The model under review builds one solid part; all positions refer to its coordinate system, in mm. A direction names the side the tool comes from. Round coordinates to 2 decimals unless told otherwise and drop trailing zeros. Write each loop counter-clockwise with the first axis right and the second up, starting at its lowest first coordinate (ties: lowest second). Pieces come first, ordered by that corner, then holes. Notation, with made-up numbers: (63, 32) - (112, 32) arc R26 cw to (112, 66) - close; hole circle Ø11 at (25.5, 22.5). An arc over 180 degrees is marked (long way). Return JSON: item names as keys, results as strings.
from build123d import *

# Parameters (mm, degrees)
EXTRUDE_1_DEPTH              = 25
EXTRUDE_2_DEPTH              = 10
HOLE_WIZARD_M8_1_D           = 15
HOLE_WIZARD_M8_1_CBORE_D     = 30
HOLE_WIZARD_M8_1_CBORE_DEPTH = 10
CUT_EXTRUDE_1_DEPTH          = 20
SKETCH_6_R                   = 35.5
EXTRUDE_3_DEPTH              = 130
SKETCH_7_R                   = 38.335
EXTRUDE_4_DEPTH              = 130
EXTRUDE_8_DEPTH              = 70
CUT_EXTRUDE_2_REACH          = 225
SKETCH_9_R                   = 20.5
CUT_EXTRUDE_3_REACH          = 212
SKETCH_10_R                  = 20.5
CHAMFER_1_SIZE               = 2


with BuildPart() as part:
    # Sketch 1 → Extrude 1 (new body)
    with BuildSketch(Plane(origin=(0, 0, 0), x_dir=(1, 0, 0), z_dir=(0, 1, 0))):
        with BuildLine():
            Line((10, 0), (190, 0))
            ThreePointArc((190, 0), (197.071067812, 2.928932188), (200, 10))
            Line((200, 10), (200, 203))
            ThreePointArc((200, 203), (197.071067812, 210.071067812), (190, 213))
            Line((190, 213), (10, 213))
            ThreePointArc((10, 213), (2.928932188, 210.071067812), (0, 203))
            Line((0, 203), (0, 10))
            ThreePointArc((0, 10), (2.928932188, 2.928932188), (10, 0))
        make_face()
    extrude(amount=EXTRUDE_1_DEPTH)

    # Sketch 2 → Extrude 2 (add)
    with BuildSketch(Plane(origin=(0, 25, 0), x_dir=(1, 0, 0), z_dir=(0, 1, 0))):
        with BuildLine():
            Line((140, 0), (190, 0))
            ThreePointArc((190, 0), (197.071067812, 2.928932188), (200, 10))
            Line((200, 10), (200, 60))
            Line((200, 60), (155, 60))
            ThreePointArc((155, 60), (144.393398282, 55.606601718), (140, 45))
            Line((140, 45), (140, 0))
        make_face()
    extrude(amount=EXTRUDE_2_DEPTH)

    # Hole Wizard M8 _ _ _ _1 (through all)
    with Locations(Plane(origin=(170, 35, -30), x_dir=(0, 0, 1), z_dir=(0, 1, 0))):
        with Locations((0, 0)):
            CounterBoreHole(HOLE_WIZARD_M8_1_D / 2, HOLE_WIZARD_M8_1_CBORE_D / 2, HOLE_WIZARD_M8_1_CBORE_DEPTH)

    # Sketch 5 → Cut-Extrude 1 (cut)
    with BuildSketch(Plane(origin=(0, 25, 0), x_dir=(1, 0, 0), z_dir=(0, 1, 0))):
        with BuildLine():
            Line((149.247641486, 146), (181, 146))
            ThreePointArc((181, 146), (188.071067812, 143.071067812), (191, 136))
            Line((191, 136), (191, 79))
            ThreePointArc((191, 79), (188.071067812, 71.928932188), (181, 69))
            Line((181, 69), (155, 69))
            ThreePointArc((155, 69), (138.029437252, 61.970562748), (131, 45))
            Line((131, 45), (131, 19))
            ThreePointArc((131, 19), (128.071067812, 11.928932188), (121, 9))
            Line((121, 9), (64, 9))
            ThreePointArc((64, 9), (56.928932188, 11.928932188), (54, 19))
            Line((54, 19), (54, 50.752358514))
            ThreePointArc((54, 50.752358514), (56.018165786, 56.776503481), (61.258064516, 60.369103795))
            ThreePointArc((61.258064516, 60.369103795), (110.610173055, 89.389826945), (139.630896205, 138.741935484))
            ThreePointArc((139.630896205, 138.741935484), (143.223496519, 143.981834214), (149.247641486, 146))
        make_face()
    extrude(amount=-CUT_EXTRUDE_1_DEPTH, mode=Mode.SUBTRACT)



with BuildPart() as body_2:
    # Sketch 6 → Extrude 3 (new body)
    with BuildSketch(Plane.XY.offset(10)):
        with Locations((37.5, 95)):
            Circle(SKETCH_6_R)
    extrude(amount=-EXTRUDE_3_DEPTH)


with BuildPart() as body_3:
    # Sketch 7 → Extrude 4 (new body)
    with BuildSketch(Plane(origin=(210, 0, 0), x_dir=(0, 0, -1), z_dir=(1, 0, 0))):
        with Locations((162.5, 95)):
            Circle(SKETCH_7_R)
    extrude(amount=-EXTRUDE_4_DEPTH)


with BuildPart() as part_1:
    add(part.part)

    add(body_2.part)  # Extrude 8 merges body 2

    add(body_3.part)  # Extrude 8 merges body 3
    # Sketch 8 → Extrude 8 (add)
    with BuildSketch(Plane(origin=(0, 25, 0), x_dir=(1, 0, 0), z_dir=(0, 1, 0))):
        with BuildLine():
            Line((30, 0), (45, 0))
            Line((45, 0), (45, 66.076951546))
            ThreePointArc((45, 66.076951546), (104.246212025, 95.753787975), (133.923048454, 155))
            Line((133.923048454, 155), (200, 155))
            Line((200, 155), (200, 170))
            Line((200, 170), (120, 170))
            ThreePointArc((120, 170), (93.639610307, 106.360389693), (30, 80))
            Line((30, 80), (30, 0))
        make_face()
    extrude(amount=EXTRUDE_8_DEPTH)

    # Sketch 9 → Cut-Extrude 2 (cut, up to next)
    with BuildSketch(Plane.XY.offset(10), mode=Mode.PRIVATE) as cut_extrude_2_sk1:
        with Locations((37.5, 95)):
            Circle(SKETCH_9_R)
    cut_extrude_2_tool1 = extrude(cut_extrude_2_sk1.sketch, amount=-CUT_EXTRUDE_2_REACH, mode=Mode.PRIVATE) & part_1.part
    add(cut_extrude_2_tool1.solids().sort_by_distance((37.5, 95, 10))[0], mode=Mode.SUBTRACT)

    # Sketch 10 → Cut-Extrude 3 (cut, up to next)
    with BuildSketch(Plane(origin=(210, 0, 0), x_dir=(0, 0, -1), z_dir=(1, 0, 0)), mode=Mode.PRIVATE) as cut_extrude_3_sk1:
        with Locations((162.5, 95)):
            Circle(SKETCH_10_R)
    cut_extrude_3_tool1 = extrude(cut_extrude_3_sk1.sketch, amount=-CUT_EXTRUDE_3_REACH, mode=Mode.PRIVATE) & part_1.part
    add(cut_extrude_3_tool1.solids().sort_by_distance((210, 95, -162.5))[0], mode=Mode.SUBTRACT)

    # Chamfer 1
    chamfer_1_edges = [part_1.edges().sort_by_distance(p)[0] for p in [
        (17, 95, 10),
        (17, 95, -120),
        (210, 95, -142),
        (80, 95, -142),
    ]]
    chamfer(chamfer_1_edges, length=CHAMFER_1_SIZE)


solid = part_1.part
(1) Add section C-C (y = 50). Write out the cut boundary in (x, z).
Filled in:
{"outline": "(30, -80) arc R90 cw to (120, -170) - (200, -170) - (200, -155) - (133.92, -155) arc R105 ccw to (45, -66.08) - (45, 0) - (30, 0) - close"}
(2) Wall thickness on line 1 (Y direction, x = 118, z = -162); line 2 (X direction, y = 8.5, z = -30); line 3 (Y direction, x = 151, z = -162.5) (3 decimals): over which ranges is each line inside the solid? List them lowest first.
Filled in:
{"line 1": "y = 0 to 25, 56.67 to 74.51, 115.49 to 133.33", "line 2": "x = 0 to 54, 131 to 162.5, 177.5 to 200", "line 3": "y = 0 to 74.5, 115.5 to 133.335"}
(3) Add section D-D (z = -162.5). Write out the cut boundary in (x, y) (3 decimals), plus the area to 3 significant figures.
Filled in:
{"outline": "(0, 0) - (200, 0) - (200, 56.665) - (210, 56.665) - (210, 72.5) - (208, 74.5) - (82, 74.5) - (80, 72.5) - (80, 56.665) - (119.687, 56.665) - (119.687, 25) - (0, 25) - close; (80, 117.5) - (82, 115.5) - (208, 115.5) - (210, 117.5) - (210, 133.335) - (80, 133.335) - close", "area": "12,200 mm2"}
(4) Add section B-B (z = -26.5). Write out the cut boundary in (x, y).
Filled in:
{"outline": "(0, 0) - (163.37, 0) - (163.37, 25) - (155.41, 25) - (155.41, 35) - (140, 35) - (140, 25) - (131, 25) - (131, 5) - (54, 5) - (54, 25) - (45, 25) - (45, 60.3) arc R35.5 ccw (long way) to (30, 60.3) - (30, 25) - (0, 25) - close; (176.63, 0) - (200, 0) - (200, 35) - (184.59, 35) - (184.59, 25) - (176.63, 25) - close; hole circle Ø41 at (37.5, 95)"}
(5) For faces 1 (the cylindrical face through (155.357, 30.07, -33.252)), 2 (the flat face through (37, 72, -120)), 3 (the cylindrical face through (103.576, 51.732, -95.089)), 4 (the flat face through (54, 15, -35)), list the 3-axis set-ups (+Z, -Z, +X, -X, +Y, -Y) from which the entire face can be reached by the end or side of a thin tool; tool diameter is ignored.
Filled in:
{"face 1": "+Y", "face 2": "-Z, -X, +Y", "face 3": "+Z, +X", "face 4": "none"}
(6) Add section A-A (x = 170). Write out the cut boundary in (y, z) (3 decimals).
Filled in:
{"outline": "(0, -213) - (25, -213) - (25, -170) - (57.406, -170) arc R38.335 ccw (long way) to (57.406, -155) - (25, -155) - (25, -146) - (5, -146) - (5, -69) - (25, -69) - (25, -60) - (35, -60) - (35, -45) - (25, -45) - (25, -37.5) - (0, -37.5) - close; (0, -22.5) - (25, -22.5) - (25, -15) - (35, -15) - (35, 0) - (0, 0) - close; hole circle Ø41 at (95, -162.5)"}
(7) Mouldability with a two-part tool opening along Z and no side actions: class faces 5 (the flat face through (156, 35, -37)), 6 (the cylindrical face through (145.88, 82.53, -146.23)), 7 (the cylindrical face through (196.99, 17.26, -2.85)), 8 (the cylindrical face through (3.01, 12.32, -210.15)) as released by +Z, released by -Z, zero draft, split by the parting line, or undercut.
Filled in:
{"face 5": "zero draft", "face 6": "undercut", "face 7": "released by +Z", "face 8": "released by -Z"}
(8) Clearance check with flat-ended pins moving along their axes: pin 1 Ø1.5 at (x, y) = (144, 96.5) entering from -Z; pin 2 Ø2 at (y, z) = (81.5, -38.5) entering from +X; pin 3 Ø5 at (y, z) = (46, -81) entering from -X. State where each tip first meets the part, or that it passes through.
Filled in:
{"pin 1": "stops at z = -200.83", "pin 2": "stops at x = 70.73", "pin 3": "stops at x = 30"}
